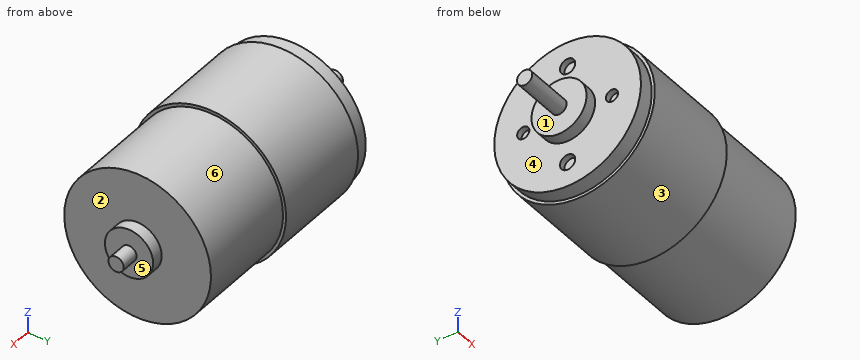
from build123d import *

# Parameters (mm, degrees)
SKETCH_2_R          = 2
SKETCH_2_R_2        = 2.5
CUT_EXTRUDE_1_DEPTH = 2


with BuildPart() as part:
    # 草图1 → 旋转1 (revolve)
    with BuildSketch(Plane(origin=(0, 0, 0), x_dir=(1, 0, 0), z_dir=(0, 1, 0)), mode=Mode.PRIVATE) as revolve_1_sk:
        Polygon((-6.743925692, 2.5), (-6.743925692, 0), (95.256074308, 0), (95.256074308, 2.5), (89.256074308, 2.5), (89.256074308, 7.88455591), (85.256074308, 7.88455591), (85.256074308, 24), (51.756074308, 24), (51.756074308, 25), (18.256074308, 25), (18.256074308, 24), (13.256074308, 24), (13.256074308, 9), (9.256074308, 9), (9.256074308, 2.5), align=None)
    revolve(revolve_1_sk.sketch.rotate(Axis((-8.123537978, 0, 0), (1, 0, 0)), 180), axis=Axis((-8.123537978, 0, 0), (1, 0, 0)))

    # 草图2 → 切除-拉伸1 (cut)
    with BuildSketch(Plane.ZY.offset(-13.256074308)):
        with Locations((0, 14.5)):
            Circle(SKETCH_2_R)
        with Locations(Location((0, -14.5, 0), (0, 0, 180))):
            Circle(SKETCH_2_R)
        with Locations((-16, 0)):
            Circle(SKETCH_2_R_2)
        with Locations(Location((16, 0, 0), (0, 0, 180))):
            Circle(SKETCH_2_R_2)
    extrude(amount=-CUT_EXTRUDE_1_DEPTH, mode=Mode.SUBTRACT)


solid = part.part
Verification items for the finished model (mm, model axes). Face numbers are marked on the shaded views. A direction names the side the tool comes from. Round coordinates to 2 decimals unless told otherwise and drop trailing zeros. Loops run counter-clockwise (first coordinate to the right, second up) from the corner with the lowest first, then second, coordinate; pieces in that order, holes last. Notation, with made-up numbers: (-16.75, 20) - (29.25, 20) arc R16 ccw to (29.25, 25) - close; hole circle Ø11 at (53.5, 78). An arc over 180 degrees is marked (long way). Write item = value, one per line.
Q1. Sectioned sample at B-B on y = 18. Record the boundary of the cut face in (x, z), plus the area to 3 significant figures.
Here are the results:
outline = (13.26, -15.87) - (18.26, -15.87) - (18.26, -17.35) - (51.76, -17.35) - (51.76, -15.87) - (85.26, -15.87) - (85.26, 15.87) - (51.76, 15.87) - (51.76, 17.35) - (18.26, 17.35) - (18.26, 15.87) - (13.26, 15.87) - close
area = 2,380 mm^2
Q2. Sectioned sample at D-D on z = 16. Record the boundary of the cut face in (x, y).
Here are the results:
outline = (13.26, -17.89) - (18.26, -17.89) - (18.26, -19.21) - (51.76, -19.21) - (51.76, -17.89) - (85.26, -17.89) - (85.26, 17.89) - (51.76, 17.89) - (51.76, 19.21) - (18.26, 19.21) - (18.26, 17.89) - (13.26, 17.89) - (13.26, 2.5) - (15.26, 2.5) - (15.26, -2.5) - (13.26, -2.5) - close
Q3. Tool access check on the marked faces 1, 2 and 3. Record the directions out of +Z, -Z, +X, -X, +Y, -Y that give a thin tool (end or side, any length) a straight path to the whole face; none if there is none.
Here are the results:
face_1 = -X
face_2 = +X
face_3 = +X, -X
Q4. Sectioned sample at C-C on x = 71. Record the boundary of the cut face in (y, z), plus the area to 3 significant figures.
Here are the results:
outline = circle Ø48 at (0, 0)
area = 1,810 mm^2
Q5. Material ranges on L1, parallel to Y at x = 14.05, z = 0; L2, parallel to X at y = 5, z = 12.5; L3, parallel to Y at x = 13, z = 0, recorded low to high.
Here are the results:
L1 = -24 to -16.5, -12.5 to 12.5, 16.5 to 24
L2 = 13.26 to 85.26
L3 = -9 to 9
Q6. Depth check by flat-ended pin: pin 1 (5 mm diameter, centred on y = 14.5, z = 0, fed in from -X); pin 2 (8 mm diameter, centred on y = 10, z = 4, fed in from +X); pin 3 (6.5 mm diameter, centred on y = 0, z = -16, fed in from +X). Enter the tip coordinate at first touch or a pass-through.
Here are the results:
pin_1 = 13.26
pin_2 = 89.26
pin_3 = 85.26
Q7. Sectioned sample at A-A on z = -17. Record the boundary of the cut face in (x, y).
Here are the results:
outline = (13.26, -16.94) - (18.26, -16.94) - (18.26, -18.33) - (51.76, -18.33) - (51.76, -16.94) - (85.26, -16.94) - (85.26, 16.94) - (51.76, 16.94) - (51.76, 18.33) - (18.26, 18.33) - (18.26, 16.94) - (13.26, 16.94) - (13.26, 2.29) - (15.26, 2.29) - (15.26, -2.29) - (13.26, -2.29) - close
Q8. Mould release check, pull along X, two halves, no side actions. Record for the marked faces 4, 5 and 6: +X half, -X half, draft (parallel to the pull), parting line (faces both ways), or undercut.
Here are the results:
face_4 = -X half
face_5 = +X half
face_6 = draft
